from build123d import *

# Parameters (mm, degrees)
SKETCH_W        = 21.85185
SKETCH_H        = 12.5
PAD_DEPTH       = 12.5
SKETCH001_R     = 1
POCKET_DEPTH    = 50
SKETCH002_R     = 1
POCKET001_DEPTH = 50


with BuildPart() as part:
    # Sketch → Pad (new body)
    with BuildSketch(Plane.XZ):
        with Locations((10.925925, 6.25)):
            Rectangle(SKETCH_W, SKETCH_H)
    extrude(amount=PAD_DEPTH)

    # Sketch001 → Pocket (cut)
    with BuildSketch(Plane.YZ):
        with Locations((-6.25, 6.25)):
            Circle(SKETCH001_R)
    extrude(amount=POCKET_DEPTH, mode=Mode.SUBTRACT)

    # Sketch002 → Pocket001 (cut)
    with BuildSketch(Plane.XZ):
        with Locations((15.60185, 6.25)):
            Circle(SKETCH002_R)
    extrude(amount=POCKET001_DEPTH, mode=Mode.SUBTRACT)


solid = part.part
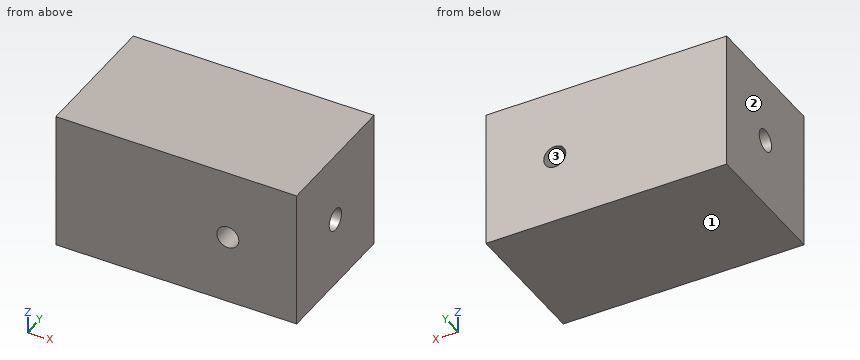
CAD build for the part. Positions are in the model's coordinates, mm. Face numbers are marked on the shaded views. Round coordinates to 2 decimals unless told otherwise and drop trailing zeros. Order: outer loops, then holes, each group sorted by start corner. A loop starts at its lowest first (then second) coordinate and runs counter-clockwise, first axis right, second up. Notation, with made-up numbers: (41, 32) -> (59, 32) arc R25 cw to (59, 48) -> close; hole circle Ø10 at (20, 13.5). An arc over 180 degrees is marked (long way). Write item = value, one per line. Start each with the question number.
(1) Cut at C-C, the plane x = 5. List the corners of the cut face in (y, z).
(2) Cut at B-B, the plane y = -6. List the corners of the cut face in (x, z).
(3) Pull direction X, two halves, no side cores. Call the marked faces 1, 2 and 3: released by +X, released by -X, zero draft, split by the parting line, or undercut.
(4) Cut at A-A, the plane z = 6.25. List the corners of the cut face in (x, y).
(5) Probe line 1 (X direction, y = -8.75, z = 6.25); line 2 (Y direction, x = 3.5, z = 6.25); line 3 (Z direction, x = 19, y = -6.25). List the from-to ranges inside material, lowest first. Write a range as [from, to].
Model answer:
q1.outline = (-12.5, 0) -> (0, 0) -> (0, 12.5) -> (-12.5, 12.5) -> close; hole circle Ø2 at (-6.25, 6.25)
q2.outline = (0, 0) -> (21.85, 0) -> (21.85, 5.28) -> (15.85, 5.28) arc R1 cw to (15.35, 5.28) -> (0, 5.28) -> close; (0, 7.22) -> (15.35, 7.22) arc R1 cw to (15.85, 7.22) -> (21.85, 7.22) -> (21.85, 12.5) -> (0, 12.5) -> close
q3.face_1 = zero draft
q3.face_2 = released by -X
q3.face_3 = undercut
q4.outline = (0, -12.5) -> (14.6, -12.5) -> (14.6, -7.25) -> (0, -7.25) -> close; (0, -5.25) -> (14.6, -5.25) -> (14.6, 0) -> (0, 0) -> close; (16.6, -12.5) -> (21.85, -12.5) -> (21.85, -7.25) -> (16.6, -7.25) -> close; (16.6, -5.25) -> (21.85, -5.25) -> (21.85, 0) -> (16.6, 0) -> close
q5.line_1 = [0, 14.6], [16.6, 21.85]
q5.line_2 = [-12.5, -7.25], [-5.25, 0]
q5.line_3 = [0, 5.25], [7.25, 12.5]
